```python
from build123d import *

# Parameters (mm, degrees)
SKETCH1_R           = 5.5499
SKETCH1_R_2         = 4.000000001
BOSS_EXTRUDE1_DEPTH = 9.525
CHAMFER1_SIZE       = 0.127


with BuildPart() as part:
    # Sketch1 → Boss-Extrude1 (new body)
    with BuildSketch(Plane.XY):
        with Locations(Location((0, 0, 0), (0, 0, 180))):
            Circle(SKETCH1_R)
        with Locations(Location((0, 0, 0), (0, 0, 180))):
            Circle(SKETCH1_R_2, mode=Mode.SUBTRACT)
    extrude(amount=BOSS_EXTRUDE1_DEPTH)

    # Chamfer1
    chamfer1_edges = [part.edges().sort_by_distance(p)[0] for p in [
        (5.5499, 0, 0),
        (5.5499, 0, 9.525),
        (4.000000001, 0, 0),
        (4.000000001, 0, 9.525),
    ]]
    chamfer(chamfer1_edges, length=CHAMFER1_SIZE)


solid = part.part
```
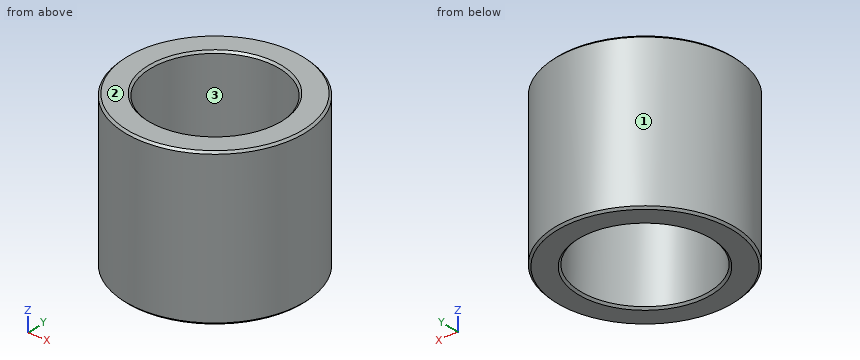
Geometry check sheet. Reference: the model listing, model coordinates, mm. Face numbers are marked on the shaded views. Coordinates: 2 decimals unless noted, no trailing zeros. Loops run counter-clockwise (first coordinate to the right, second up) from the corner with the lowest first, then second, coordinate; pieces in that order, holes last. Notation, with made-up numbers: (9, -20) -> (44, -20) arc R30 cw to (44, 19) -> close; hole circle Ø4 at (-37.5, -25). An arc over 180 degrees is marked (long way). Put each result on its own line as item: value.
1) Gauge pin test, flat ends, axial feed: pin 1 Ø1.5 at (x, z) = (-3, 2) entering from +Y; pin 2 Ø3 at (y, z) = (4.5, 3.5) entering from +X; pin 3 Ø1.5 at (x, z) = (3.5, 3.5) entering from -Y. Record the tip position at first contact, or that the pin passes through.
Result set:
pin 1: stops at y = 5.07
pin 2: stops at x = 4.67
pin 3: stops at y = -4.82
2) Cross-section at C-C on z = 6.5. Record the boundary of the cut face in (x, y).
Result set:
outline: circle Ø11.1 at (0, 0); hole circle Ø8 at (0, 0)
3) Thickness scan on line 1 (Y direction, x = 0, z = 2.5); line 2 (Y direction, x = 2.75, z = 5.5). Record the ranges inside material, lowest first.
Result set:
line 1: y = -5.55 to -4, 4 to 5.55
line 2: y = -4.82 to -2.9, 2.9 to 4.82
4) Cross-section at A-A on x = 0. Record the boundary of the cut face in (y, z) (3 decimals).
Result set:
outline: (-5.55, 0.127) -> (-5.423, 0) -> (-4.127, 0) -> (-4, 0.127) -> (-4, 9.398) -> (-4.127, 9.525) -> (-5.423, 9.525) -> (-5.55, 9.398) -> close; (4, 0.127) -> (4.127, 0) -> (5.423, 0) -> (5.55, 0.127) -> (5.55, 9.398) -> (5.423, 9.525) -> (4.127, 9.525) -> (4, 9.398) -> close
5) Release check for a two-part mould opening along X. For the marked faces 1, 2 and 3 record: released by +X, released by -X, zero draft, split by the parting line, or undercut.
Result set:
face 1: split by the parting line
face 2: zero draft
face 3: undercut
